The drawing under review shows one solid part. Ordinate dimensions are in mm from its lowest x, y, z. Coordinates: 2 decimals unless noted, no trailing zeros. Write each loop counter-clockwise with the first axis right and the second up, starting at its lowest first coordinate (ties: lowest second). Pieces come first, ordered by that corner, then holes.
1) We need section B-B on y = 3.5. Write out the cut boundary in (x, z).
2) We need section C-C on x = 150. Write out the cut boundary in (y, z).
3) To check wall thickness, follow line 1 along Z through (x, y) = (50, 4); line 2 along Z through (x, y) = (154.5, 8.75). State the ranges of each line that lie inside material, in increasing order.
4) We need section A-A on z = 150. Write out the cut boundary in (x, y).
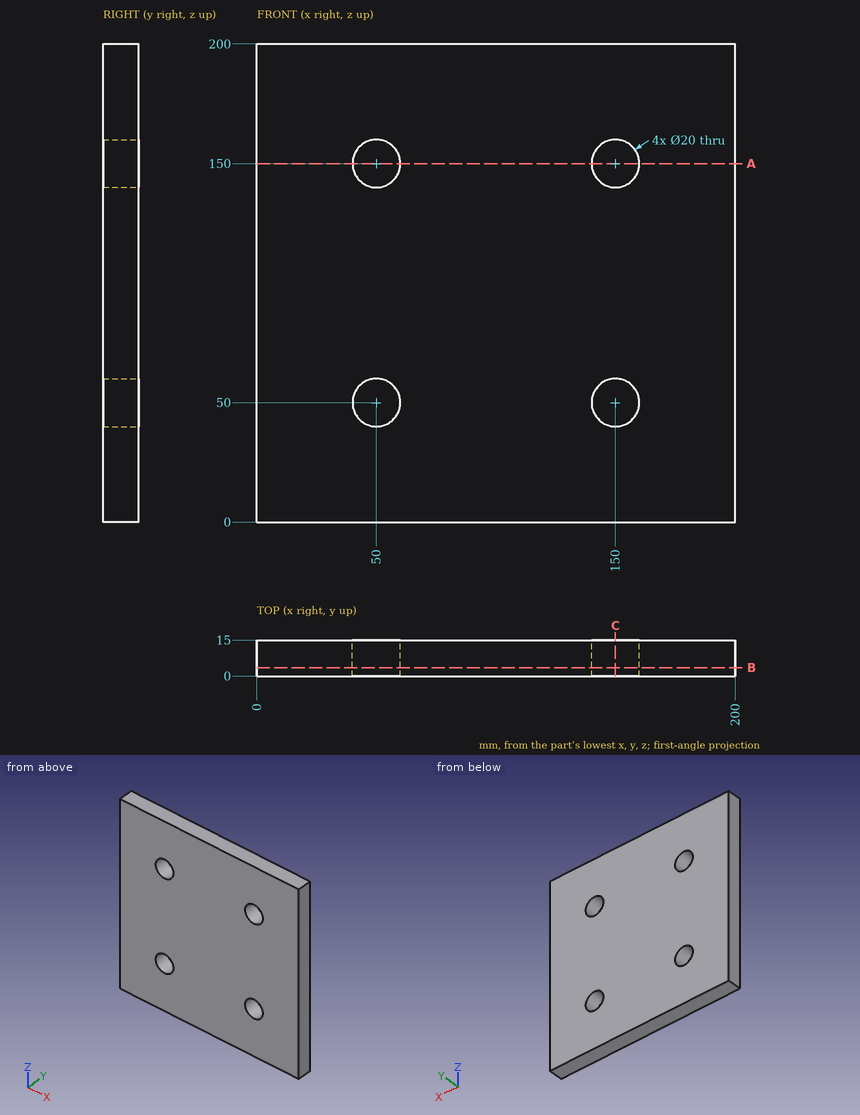
Result:
1. outline: (0, 0) - (200, 0) - (200, 200) - (0, 200) - close; hole circle Ø20 at (50, 50); hole circle Ø20 at (50, 150); hole circle Ø20 at (150, 50); hole circle Ø20 at (150, 150)
2. outline: (0, 0) - (15, 0) - (15, 40) - (0, 40) - close; (0, 60) - (15, 60) - (15, 140) - (0, 140) - close; (0, 160) - (15, 160) - (15, 200) - (0, 200) - close
3. line 1: z = 0 to 40, 60 to 140, 160 to 200
3. line 2: z = 0 to 41.07, 58.93 to 141.07, 158.93 to 200
4. outline: (0, 0) - (40, 0) - (40, 15) - (0, 15) - close; (60, 0) - (140, 0) - (140, 15) - (60, 15) - close; (160, 0) - (200, 0) - (200, 15) - (160, 15) - close
